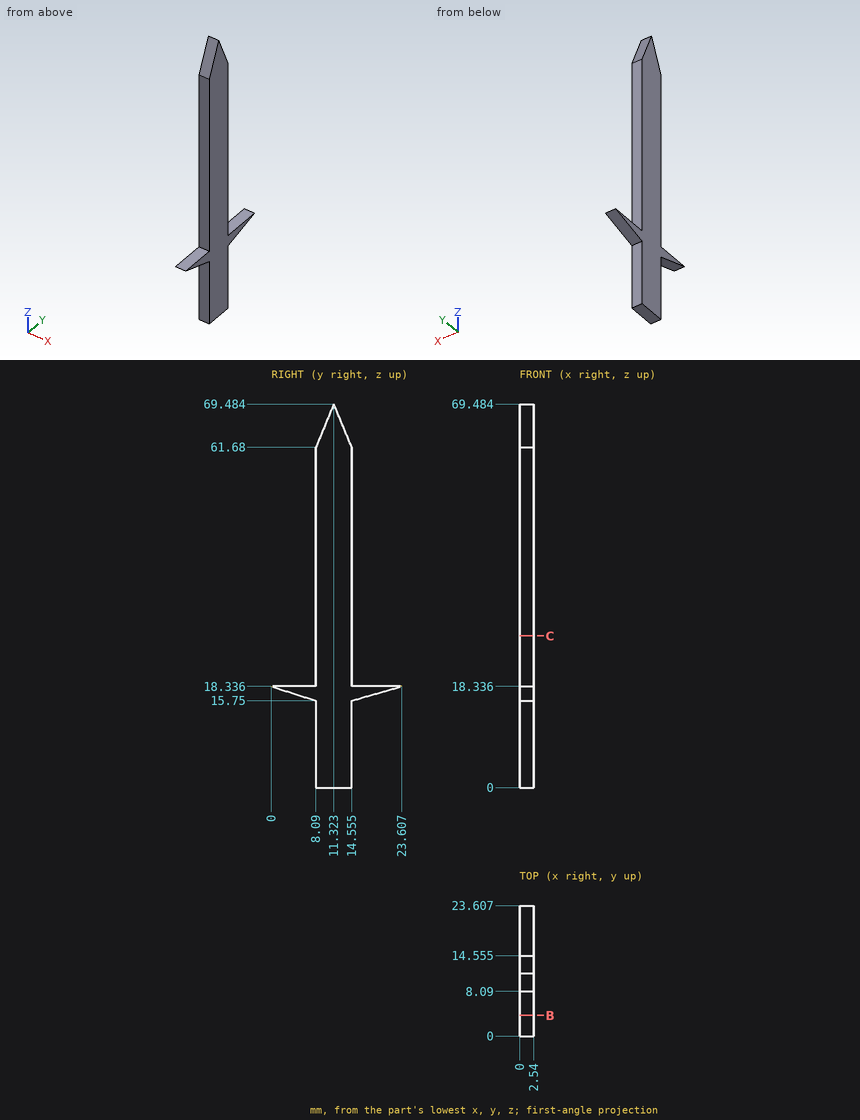
Geometry: see drawing. Coordinates: mm, zero at the bounding-box minimum. Round coordinates to 2 decimals unless told otherwise and drop trailing zeros. Loops run counter-clockwise (first coordinate to the right, second up) from the corner with the lowest first, then second, coordinate; pieces in that order, holes last.
(1) Contact query for flat-ended pins moving along their axis: pin 1 Ø1.3 at (x, z) = (1, 46.5) entering from +Y (1 decimal); pin 2 Ø10 at (y, z) = (2.5, 43) entering from +X; pin 3 Ø0.8 at (x, y) = (1, 18) entering from +Z. Output: stop coordinate, or through.
From the geometry:
pin 1: stops at y = 14.6
pin 2: passes through
pin 3: stops at z = 18.34
(2) Section query C-C (z = 27.5). Output: boundary loops of the cut face in (x, y) (1 decimal), and give its area (3 significant figures).
From the geometry:
outline: (0, 8.1) - (2.5, 8.1) - (2.5, 14.6) - (0, 14.6) - close
area: 16.4 mm2
(3) Material intervals for probe 1 along Y at (x, z) = (1.9, 38) (1 decimal); probe 2 along Z at (x, y) = (1.9, 16.75); probe 3 along Z at (x, y) = (1.1, 5), sorted ascending.
From the geometry:
probe 1: y = 8.1 to 14.6
probe 2: z = 16.38 to 18.34
probe 3: z = 16.74 to 18.34
(4) Section query B-B (y = 3.75). Output: boundary loops of the cut face in (x, z).
From the geometry:
outline: (0, 17.14) - (2.54, 17.14) - (2.54, 18.34) - (0, 18.34) - close
